Source: CAD feature listing. Evaluate the final solid. Frame: model axes, mm. A direction names the side the tool comes from. Give positions to 0.01 mm unless a question says otherwise; leave off trailing zeros. Use CSV: the item, a comma, the result in double quotes.
```python
from build123d import *

# Parameters (mm, degrees)
F2_R     = 25.4
F3_SCALE = 1.6


with BuildPart() as f1:
    # F0 (on Front) → F1 (revolve)
    with BuildSketch(Plane.XZ):
        Polygon((111.125, 222.25), (111.125, 241.3), (-111.125, 241.3), (-111.125, 222.25), (-29.2621003771, 222.25), (-5.1864683628, 222.25), align=None)
        Polygon((-98.425, 101.6), (-5.1864683628, 222.25), (-29.2621003771, 222.25), (-122.5006320143, 101.6), align=None)
        Polygon((-28.575, 101.6), (-98.425, 101.6), (-122.5006320143, 101.6), (-168.275, 101.6), (-168.275, 31.75), (-28.575, 31.75), align=None)
    revolve(axis=Axis((-5.1864683628, 0, 0), (1, 0, 0)))

    # F2
    f2_edges = [f1.edges().sort_by_distance(p)[0] for p in [
        (-98.425, 0, -101.6),
        (-5.186468, 0, -222.25),
        (-51.805734, 0, 161.925),
        (-29.2621, 0, -222.25),
        (-122.500632, 0, -101.6),
        (-75.881366, 0, 161.925),
    ]]
    fillet(f2_edges, radius=F2_R)


with BuildPart() as f1_1:
    # F3: moved
    add(f1.part.scale(F3_SCALE))


solid = f1_1.part
```
Item 1: Set-up query: faces 1 (the cylindrical face through (-243, -49, 155)), 2 (the flat face through (-269.24, -38, 34)), 3 (the flat face through (-45.72, -38, -34)). Return all of +Z, -Z, +X, -X, +Y, -Y with unobstructed straight access to the full face (end or side cutting, diameter ignored); none if empty.
Filled in:
face 1,"-X"
face 2,"+Z, -Z, -X, +Y, -Y"
face 3,"+X"
Item 2: First-contact query: pin 1 (2 mm diameter, centred on y = 84.5, z = 261, fed in from -X); pin 2 (12 mm diameter, centred on x = -212.5, y = -79, fed in from -Z); pin 3 (12 mm diameter, centred on y = -99, z = -108, fed in from +X). Flat tips, straight axial feed; report the tip coordinate or a pass-through.
Filled in:
pin 1,"stops at x = -110.39"
pin 2,"stops at z = -145.49"
pin 3,"stops at x = -45.72"
Item 3: Material intervals for line 1 (Y direction, x = -153, z = 0); line 2 (Z direction, x = -156, y = 0); line 3 (Z direction, x = -148, y = 0), sorted ascending. Write a range as from..to.
Filled in:
line 1,"y = -386.08..-355.6, -218.2..-50.8, 50.8..218.2, 355.6..386.08"
line 2,"z = -386.08..-355.6, -214.32..-50.8, 50.8..214.32, 355.6..386.08"
line 3,"z = -386.08..-355.6, -224.67..-50.8, 50.8..224.67, 355.6..386.08"
